```python
from build123d import *

# Parameters (mm, degrees)
F1_DEPTH = 15
F2_R     = 2.25
F3_DEPTH = 25
F5_R     = 2.25
F6_DEPTH = 1.5
F7_W     = 15
F7_H     = 15
F7_R     = 2
F8_DEPTH = 5
F9_R     = 1
F10_SIZE = 2


with BuildPart() as f1:
    # F0 (on Front) → F1 (new body)
    with BuildSketch(Plane.XZ):
        Polygon((-57.5, -25.5), (-57.5, 25.5), (-8.5, 25.5), (-2.5, 25.5), (-2.5, 41.5), (-8.5, 41.5), (-8.5, 29.5), (-61.5, 29.5), (-61.5, -29.5), (61.5, -29.5), (61.5, 29.5), (8.5, 29.5), (8.5, 41.5), (2.5, 41.5), (2.5, 25.5), (8.5, 25.5), (57.5, 25.5), (57.5, -25.5), align=None)
    extrude(amount=F1_DEPTH)

    # F2 (on face) → F3 (cut)
    with BuildSketch(Plane.YZ.offset(8.5)):
        with Locations((-7.5, 35.5)):
            Circle(F2_R)
    extrude(amount=-F3_DEPTH, mode=Mode.SUBTRACT)

    # F5 (on face) → F6 (cut)
    with BuildSketch(Plane(origin=(-8.5, 0, 0), x_dir=(0, -1, 0), z_dir=(-1, 0, 0))):
        Polygon((9.45799692, 31.9645252943), (11.5408093696, 35.4279377204), (9.5828124496, 38.9634124261), (5.54200308, 39.0354747057), (3.4591906304, 35.5720622796), (5.4171875504, 32.0365875739), align=None)
        with Locations((7.5, 35.5)):
            Circle(F5_R, mode=Mode.SUBTRACT)
    extrude(amount=-F6_DEPTH, mode=Mode.SUBTRACT)

    # F7 (on face) → F8 (join)
    with BuildSketch(Plane(origin=(0, 0, -29.5), x_dir=(1, 0, 0), z_dir=(0, 0, -1))):
        with Locations((-69, 7.5)):
            Rectangle(F7_W, F7_H)
        with Locations((-69, 7.5)):
            Circle(F7_R, mode=Mode.SUBTRACT)
        with Locations((69, 7.5)):
            Rectangle(F7_W, F7_H)
        with Locations((69, 7.5)):
            Circle(F7_R, mode=Mode.SUBTRACT)
    extrude(amount=-F8_DEPTH)

    # F9
    f9_edges = [f1.edges().sort_by_distance(p)[0] for p in [
        (30, 0, 25.5),
        (57.5, 0, 0),
        (-30, 0, 25.5),
        (-57.5, 0, 0),
        (0, 0, -25.5),
        (-30, -15, 25.5),
        (30, -15, 25.5),
        (-57.5, -15, 0),
        (0, -15, -25.5),
        (57.5, -15, 0),
        (-69, -15, -24.5),
        (-76.5, -7.5, -24.5),
        (-69, 0, -24.5),
        (69, 0, -24.5),
        (76.5, -7.5, -24.5),
        (69, -15, -24.5),
        (61.5, -7.5, -24.5),
        (-61.5, -7.5, -24.5),
        (-35, -15, 29.5),
        (-35, 0, 29.5),
        (35, 0, 29.5),
        (8.5, -7.5, 29.5),
        (-8.5, -7.5, 29.5),
        (-8.5, -4.500597, 37.303768),
        (-8.5, -15, 35.5),
        (-8.5, 0, 35.5),
        (-8.5, -7.5, 41.5),
        (8.5, -7.5, 41.5),
        (8.5, -15, 35.5),
        (35, -15, 29.5),
        (61.5, -7.5, 29.5),
        (-61.5, -7.5, 29.5),
        (5.5, 0, 41.5),
        (-5.5, 0, 41.5),
        (-5.5, -15, 41.5),
        (5.5, -15, 41.5),
        (-61.5, -15, 2.5),
        (61.5, -15, 2.5),
        (8.5, 0, 35.5),
        (61.5, 0, 2.5),
        (-61.5, 0, 2.5),
    ]]
    fillet(f9_edges, radius=F9_R)

    # F10
    f10_edges = [f1.edges().sort_by_distance(p)[0] for p in [
        (67, -7.5, -24.5),
        (-71, -7.5, -24.5),
    ]]
    chamfer(f10_edges, length=F10_SIZE)


solid = f1.part
```
Geometry check sheet. Reference: the model listing, model coordinates, mm. A direction names the side the tool comes from. Coordinates: 2 decimals unless noted, no trailing zeros. Loops run counter-clockwise (first coordinate to the right, second up) from the corner with the lowest first, then second, coordinate; pieces in that order, holes last.
Item 1: Sectioned sample at B-B, the plane z = 23.5. Record the boundary of the cut face in (x, y), then the cut area to 3 significant figures.
Item 2: Release check for a two-part mould opening along Y. For faces 1 (the face through (57.5, -7, 0)), 2 (the face through (69, -5, -26)) record: released by +Y, released by -Y, zero draft, split by the parting line, or undercut.
Item 3: Sectioned sample at D-D, the plane y = -7.5. Count the separate pieces of the cut face and the enclosed holes in it, then the cut area to 3 significant figures.
Item 4: Sectioned sample at C-C, the plane x = 30. Record the boundary of the cut face in (y, z).
Item 5: Sectioned sample at A-A, the plane x = 69. Record the boundary of the cut face in (y, z).
Item 6: Go/stop test with flat-tipped pins: pin 1 Ø4 at (y, z) = (-5, -3.5) entering from +X; pin 2 Ø12 at (x, z) = (-56.5, -11.5) entering from -Y; pin 3 Ø3.5 at (y, z) = (-6.5, 34) entering from -X; pin 4 Ø4 at (x, y) = (-30, -5) entering from +Z. Record where each tip stops, or that it passes through.
Item 7: Thickness scan on line 1 (X direction, y = -7.5, z = -28); line 2 (Z direction, x = -4.7, y = -7.5); line 3 (Z direction, x = 55, y = -9). Record the ranges inside material, lowest first.
Item 8: Access from +Z, -Z, +X, -X, +Y, -Y to the whole of each face (thin tool, end or side, straight path). Record for faces 3 (the face through (-7, -7, 38)), 4 (the face through (-61.5, -7, 3)), 5 (the face through (-57.5, -7, 0)).
Check result:
1. outline: (-61.5, -14) arc R1 ccw to (-60.5, -15) - (-58.5, -15) arc R1 ccw to (-57.5, -14) - (-57.5, -1) arc R1 ccw to (-58.5, 0) - (-60.5, 0) arc R1 ccw to (-61.5, -1) - close; (57.5, -14) arc R1 ccw to (58.5, -15) - (60.5, -15) arc R1 ccw to (61.5, -14) - (61.5, -1) arc R1 ccw to (60.5, 0) - (58.5, 0) arc R1 ccw to (57.5, -1) - close
1. area: 118 mm2
2. face 1: zero draft
2. face 2: undercut
3. separate pieces: 5
3. enclosed holes: 0
3. area: 1,560 mm2
4. outline: (-15, -29.5) - (0, -29.5) - (0, -26.5) arc R1 ccw to (-1, -25.5) - (-14, -25.5) arc R1 ccw to (-15, -26.5) - close; (-15, 26.5) arc R1 ccw to (-14, 25.5) - (-1, 25.5) arc R1 ccw to (0, 26.5) - (0, 28.5) arc R1 ccw to (-1, 29.5) - (-14, 29.5) arc R1 ccw to (-15, 28.5) - close
5. outline: (-15, -29.5) - (-9.5, -29.5) - (-9.5, -26.5) - (-11.5, -24.5) - (-14, -24.5) arc R1 ccw to (-15, -25.5) - close; (-5.5, -29.5) - (0, -29.5) - (0, -25.5) arc R1 ccw to (-1, -24.5) - (-3.5, -24.5) - (-5.5, -26.5) - close
6. pin 1: stops at x = 61.5
6. pin 2: stops at y = -15
6. pin 3: stops at x = -7
6. pin 4: stops at z = 29.5
7. line 1: x = -76.5 to -71, -67 to 67, 71 to 76.5
7. line 2: z = -29.5 to -25.5, 25.5 to 33.25, 37.75 to 41.5
7. line 3: z = -29.5 to -25.5, 25.5 to 29.5
8. face 3: -X
8. face 4: +Z, -X, +Y, -Y
8. face 5: +Y, -Y
